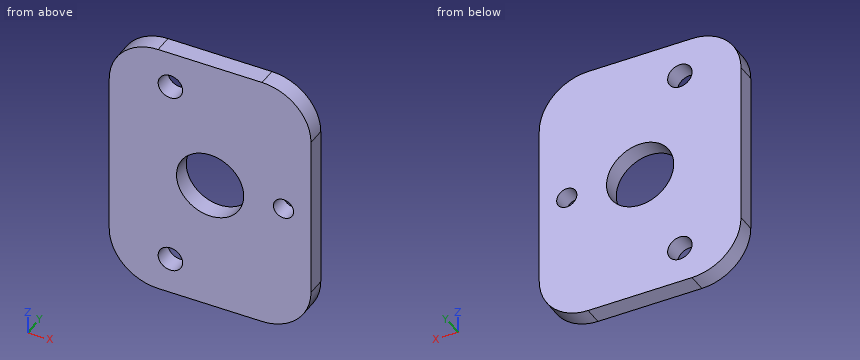
from build123d import *

# Parameters (mm, degrees)
SKETCH1_W           = 33
SKETCH1_H           = 43
SKETCH1_R           = 5.5
BOSS_EXTRUDE1_DEPTH = 3
SKETCH2_R           = 2
SKETCH2_R_2         = 1.65
CUT_EXTRUDE1_DEPTH  = 10
FILLET1_R           = 8


with BuildPart() as part:
    # Sketch1 → Boss-Extrude1 (new body)
    with BuildSketch(Plane(origin=(0, 0, 0), x_dir=(1, 0, 0), z_dir=(0, 1, 0))):
        Rectangle(SKETCH1_W, SKETCH1_H)
        with Locations(Location((0, 0, 0), (0, 0, 270))):
            Circle(SKETCH1_R, mode=Mode.SUBTRACT)
    extrude(amount=BOSS_EXTRUDE1_DEPTH)

    # Sketch2 → Cut-Extrude1 (cut)
    with BuildSketch(Plane(origin=(0, 3, 0), x_dir=(1, 0, 0), z_dir=(0, 1, 0))):
        with Locations(Location((-6.5, 15.5, 0), (0, 0, 270))):
            Circle(SKETCH2_R)
        with Locations(Location((-6.5, -15.5, 0), (0, 0, 270))):
            Circle(SKETCH2_R)
        with Locations(Location((12, 0, 0), (0, 0, 270))):
            Circle(SKETCH2_R_2)
    extrude(amount=-CUT_EXTRUDE1_DEPTH, mode=Mode.SUBTRACT)

    # Fillet1
    fillet1_edges = [part.edges().sort_by_distance(p)[0] for p in [
        (16.5, 1.5, 21.5),
        (-16.5, 1.5, 21.5),
        (-16.5, 1.5, -21.5),
        (16.5, 1.5, -21.5),
    ]]
    fillet(fillet1_edges, radius=FILLET1_R)


solid = part.part
Verification items for the finished model (mm, model axes). Coordinates: 2 decimals unless noted, no trailing zeros. Order: outer loops, then holes, each group sorted by start corner. A loop starts at its lowest first (then second) coordinate and runs counter-clockwise, first axis right, second up.
1. Sectioned sample at A-A, the plane z = 0. Record the cut outline in (x, y), and give its area (3 significant figures).
Results found:
outline: (-16.5, 0) - (-5.5, 0) - (-5.5, 3) - (-16.5, 3) - close; (5.5, 0) - (10.35, 0) - (10.35, 3) - (5.5, 3) - close; (13.65, 0) - (16.5, 0) - (16.5, 3) - (13.65, 3) - close
area: 56.1 mm2
2. Scan lines: line 1 (X direction, y = 0.8, z = 0); line 2 (X direction, y = 1, z = -1.5); line 3 (Z direction, x = -2.5, y = 1.8). Record each from-to range of solid material in increasing order.
Results found:
line 1: x = -16.5 to -5.5, 5.5 to 10.35, 13.65 to 16.5
line 2: x = -16.5 to -5.29, 5.29 to 11.31, 12.69 to 16.5
line 3: z = -21.5 to -4.9, 4.9 to 21.5
3. Sectioned sample at B-B, the plane x = -6.5. Record the cut outline in (y, z).
Results found:
outline: (0, -21.5) - (3, -21.5) - (3, -17.5) - (0, -17.5) - close; (0, -13.5) - (3, -13.5) - (3, 13.5) - (0, 13.5) - close; (0, 17.5) - (3, 17.5) - (3, 21.5) - (0, 21.5) - close
4. Sectioned sample at D-D, the plane x = 0. Record the cut outline in (y, z).
Results found:
outline: (0, -21.5) - (3, -21.5) - (3, -5.5) - (0, -5.5) - close; (0, 5.5) - (3, 5.5) - (3, 21.5) - (0, 21.5) - close
5. Sectioned sample at C-C, the plane z = 15.5. Record the cut outline in (x, y).
Results found:
outline: (-16.25, 0) - (-8.5, 0) - (-8.5, 3) - (-16.25, 3) - close; (-4.5, 0) - (16.25, 0) - (16.25, 3) - (-4.5, 3) - close
